```python
from build123d import *

# Parameters (mm, degrees)
SKETCH1_W                       = 40
SKETCH1_H                       = 25
BOSS_EXTRUDE1_DEPTH             = 10
SKETCH2_W                       = 29
SKETCH2_H                       = 11.6
CUT_EXTRUDE1_DEPTH              = 0.1
SKETCH4_W                       = 38.2
SKETCH4_H                       = 23.2
BOSS_EXTRUDE2_DEPTH             = 4
SKETCH5_W                       = 36
SKETCH5_H                       = 21
BOSS_EXTRUDE3_DEPTH             = 2.4
BOSS_EXTRUDE5_DEPTH             = 2.8
BOSS_EXTRUDE5_DIRECTION_2_REACH = 34.876
FILLET1_R                       = 2


with BuildPart() as part:
    # Sketch1 → Boss-Extrude1 (new body)
    with BuildSketch(Plane.XY):
        Rectangle(SKETCH1_W, SKETCH1_H)
    extrude(amount=BOSS_EXTRUDE1_DEPTH)

    # Sketch2 → Cut-Extrude1 (cut)
    with BuildSketch(Plane.XY.offset(10)):
        with Locations((0, 2.3)):
            Rectangle(SKETCH2_W, SKETCH2_H)
    extrude(amount=-CUT_EXTRUDE1_DEPTH, mode=Mode.SUBTRACT)

    # Sketch4 → Boss-Extrude2 (add)
    with BuildSketch(Plane(origin=(0, 0, 0), x_dir=(-1, 0, 0), z_dir=(0, 0, -1))):
        Rectangle(SKETCH4_W, SKETCH4_H)
    extrude(amount=BOSS_EXTRUDE2_DEPTH)

    # Sketch5 → Boss-Extrude3 (add)
    with BuildSketch(Plane(origin=(0, 0, -4), x_dir=(-1, 0, 0), z_dir=(0, 0, -1))):
        Rectangle(SKETCH5_W, SKETCH5_H)
    extrude(amount=BOSS_EXTRUDE3_DEPTH)

    # Sketch7 → Boss-Extrude5 (add)
    with BuildSketch(Plane.XZ.offset(11.6)):
        Polygon((14.5, 0), (9.5, -5), (-4.5, -5), (-9.5, 0), align=None)
    extrude(amount=BOSS_EXTRUDE5_DEPTH)

    # Boss-Extrude5 direction 2: up to this face of the body (flat: up to its plane)
    boss_extrude5_direction_2_end = Plane(part.part.faces().sort_by_distance((0, -10.5, -5.2))[0])
    # Sketch7 → Boss-Extrude5 direction 2 (add, up to the picked face)
    with BuildSketch(Plane.XZ.offset(11.6), mode=Mode.PRIVATE) as boss_extrude5_direction_2_sk1:
        Polygon((14.5, 0), (9.5, -5), (-4.5, -5), (-9.5, 0), align=None)
    boss_extrude5_direction_2_tool1 = split(extrude(boss_extrude5_direction_2_sk1.sketch, amount=-BOSS_EXTRUDE5_DIRECTION_2_REACH, mode=Mode.PRIVATE), bisect_by=boss_extrude5_direction_2_end, keep=Keep.BOTH, mode=Mode.PRIVATE)
    add(boss_extrude5_direction_2_tool1.solids().sort_by(Axis((2.5, -11.6, -2.280702), (0, 1, 0)))[0])

    # Fillet1
    # the kernel refuses this fillet: 2 mm, written as the material it takes off along each edge
    with BuildSketch(Plane(origin=(-14.493746089, -14.4, 0), x_dir=(0, 1, 0), z_dir=(1, 0, 0))) as fillet1_piece_1:
        with BuildLine():
            CenterArc((2, -1.997498436), FILLET1_R, 92.865983983, 87.134016017)
            Line((0, -1.997498436), (-0.04, -1.997498436))
            Line((-0.04, -1.997498436), (-0.04, 0))
            Line((-0.04, 0), (0, 0.04))
            ThreePointArc((0, 0.04), (0.95, 0.04), (1.898, 0.039949969))
            Line((1.898, 0.039949969), (1.9, 0))
        make_face()
    extrude(amount=33.987492178, mode=Mode.SUBTRACT)
    with BuildSketch(Plane(origin=(14.5, -14.4, -5), x_dir=(0, 1, 0), z_dir=(-1, 0, 0))) as fillet1_piece_2:
        with BuildLine():
            CenterArc((FILLET1_R, -FILLET1_R), FILLET1_R, 90, 90)
            Line((0, -FILLET1_R), (-FILLET1_R * 0.02, -FILLET1_R))
            Line((-FILLET1_R * 0.02, -FILLET1_R), (-FILLET1_R * 0.02, FILLET1_R * 0.02))
            Line((-FILLET1_R * 0.02, FILLET1_R * 0.02), (FILLET1_R, FILLET1_R * 0.02))
            Line((FILLET1_R, FILLET1_R * 0.02), (FILLET1_R, 0))
        make_face()
    extrude(amount=24, mode=Mode.SUBTRACT)


solid = part.part
```
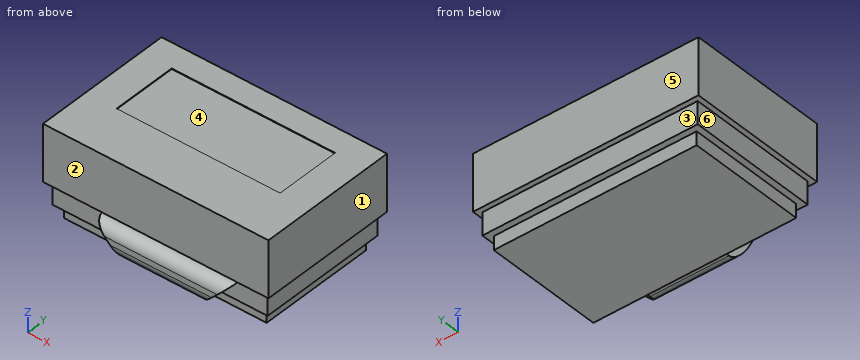
Could you check a few things on this model? Use its own coordinates, in mm. Face numbers are marked on the shaded views. A direction names the side the tool comes from. Round coordinates to 2 decimals unless told otherwise and drop trailing zeros. Write each loop counter-clockwise with the first axis right and the second up, starting at its lowest first coordinate (ties: lowest second). Pieces come first, ordered by that corner, then holes. Notation, with made-up numbers: M -17,61 L 4,61 A24 cw 4,72 Z; hole C 62,-4 d2. An arc over 180 degrees is marked long. Write each question's results on one line, items separated by ' | '. Start each with the question number.
1. Imagine slicing it at D-D on x = -11. List the corners of the cut face in (y, z) for me.
2. On a 3-axis mill with a long thin cutter (end or side, diameter ignored), from which of +Z, -Z, +X, -X, +Y, -Y can I reach the whole of each face in a straight line? I mean the marked faces 1, 2 and 3. Say none if no direction works.
3. Thinking about a two-plate mould opening in X: for the marked faces 4, 5 and 6, which applies, +X half, -X half, draft (parallel to the pull), parting line (faces both ways), or undercut?
4. Imagine slicing it at B-B on x = 9. List the corners of the cut face in (y, z) for me, and give its area (3 significant figures).
5. I'm going to push flat-ended pins straight in: pin 1 Ø4.5 at (y, z) = (-3.5, -2.5) entering from -X; pin 2 Ø1.2 at (y, z) = (-3, -1) entering from +X; pin 3 Ø1.9 at (y, z) = (0, -5) entering from -X. Where does each tip first touch, or does it pass through?
6. Imagine slicing it at C-C on z = -0.75. List the corners of the cut face in (x, y) for me, and give its area (3 significant figures).
7. I need wall thicknesses on L1, parallel to X at y = 5, z = -2.75; L2, parallel to Z at x = -4, y = 4; L3, parallel to Y at x = 12, z = -5.25. Which ranges of each line are inside material? Lowest first, please. Write a range as from..to.
8. Imagine slicing it at A-A on y = -8.25. List the corners of the cut face in (x, z) for me.
Result sheet:
1) outline: M -12.5,0 L -11.6,0 L -11.6,-4 L -10.5,-4 L -10.5,-6.4 L 10.5,-6.4 L 10.5,-4 L 11.6,-4 L 11.6,0 L 12.5,0 L 12.5,10 L 8.1,10 L 8.1,9.9 L -3.5,9.9 L -3.5,10 L -12.5,10 Z
2) face 1: +Z, -Z, +X, +Y, -Y | face 2: +Z, +X, -X, -Y | face 3: -Z, +X, -X, +Y
3) face 4: undercut | face 5: draft | face 6: -X half
4) outline: M -14.4,-3 A2 ccw -12.4,-5 L -10.5,-5 L -10.5,-6.4 L 10.5,-6.4 L 10.5,-4 L 11.6,-4 L 11.6,0 L 12.5,0 L 12.5,10 L 8.1,10 L 8.1,9.9 L -3.5,9.9 L -3.5,10 L -12.5,10 L -12.5,0 A2 ccw -14.4,-2 Z | area: 405 mm^2
5) pin 1: stops at x = -19.1 | pin 2: stops at x = 19.1 | pin 3: stops at x = -18
6) outline: M -19.1,-11.6 L -8.75,-11.6 L -8.75,-13.96 L 13.75,-13.96 L 13.75,-11.6 L 19.1,-11.6 L 19.1,11.6 L -19.1,11.6 Z | area: 939 mm^2
7) L1: x = -19.1..19.1 | L2: z = -6.4..9.9 | L3: y = -10.5..10.5
8) outline: M -20,0 L -19.1,0 L -19.1,-4 L -18,-4 L -18,-6.4 L 18,-6.4 L 18,-4 L 19.1,-4 L 19.1,0 L 20,0 L 20,10 L -20,10 Z
